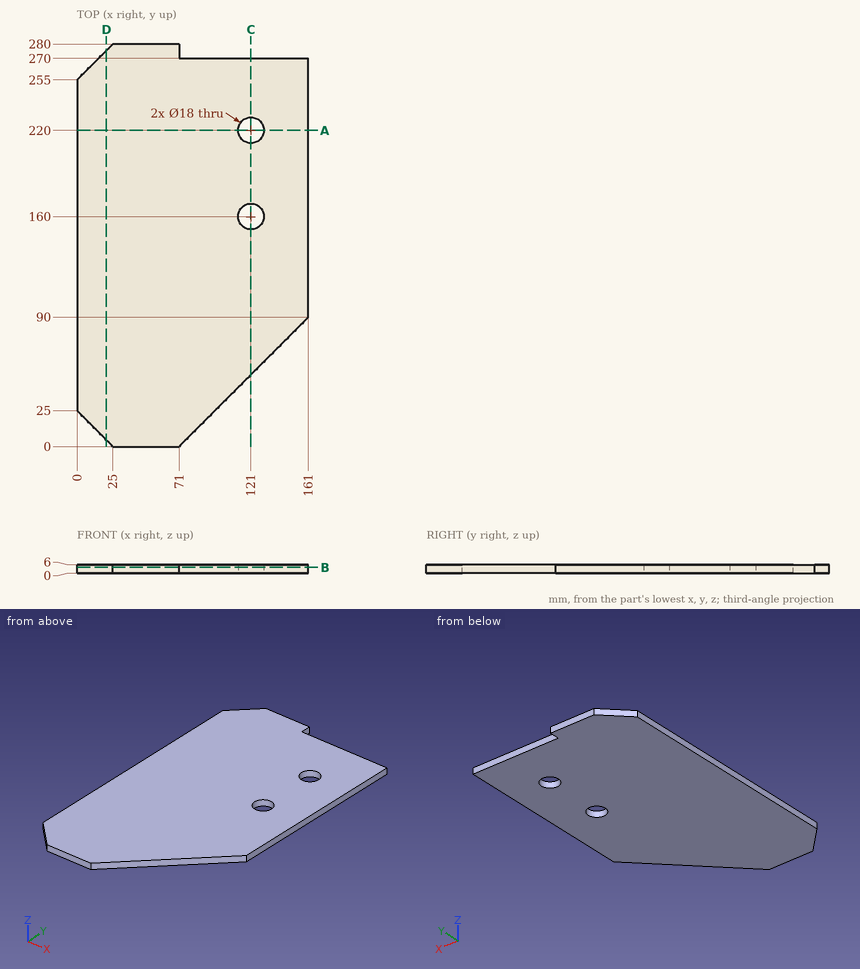
Job drawing, mm, ordinate dimensions from the low corner. One solid piece. Coordinates: 2 decimals unless noted, no trailing zeros. Loops run counter-clockwise (first coordinate to the right, second up) from the corner with the lowest first, then second, coordinate; pieces in that order, holes last. Notation, with made-up numbers: (-2, 56.5) - (31, 56.5) arc R19 ccw to (31, 83.5) - close; hole circle Ø1 at (34.5, -27). An arc over 180 degrees is marked (long way). Write item = value, one per line. Start each with the question number.
Q1. Cut at C-C, the plane x = 121. List the corners of the cut face in (y, z).
Q2. Flat gauge pins, fed straight in: pin 1 Ø10 at (x, y) = (75.5, 71.5) entering from -Z; pin 2 Ø3 at (x, z) = (145, 3) entering from +Y; pin 3 Ø14.5 at (x, y) = (121, 160) entering from +Z. Where does each tip first touch, or does it go through?
Q3. Cut at B-B, the plane z = 3.95. List the corners of the cut face in (x, y), then the cut area to 3 significant figures.
Q4. Cut at D-D, the plane x = 20.5. List the corners of the cut face in (y, z).
Q5. Cut at A-A, the plane y = 220. List the corners of the cut face in (x, z), then the cut area to 3 significant figures.
Q6. Drill centre lines: L1, parallel to X at y = 220, z = 1.9; L2, parallel to Y at x = 119, z = 3.25; L3, parallel to Y at x = 121, z = 2.3. Where is each one in solid material? Low to high.
Computed:
q1.outline = (50, 0) - (151, 0) - (151, 6) - (50, 6) - close; (169, 0) - (211, 0) - (211, 6) - (169, 6) - close; (229, 0) - (270, 0) - (270, 6) - (229, 6) - close
q2.pin_1 = 0
q2.pin_2 = 270
q2.pin_3 = through
q3.outline = (0, 25) - (25, 0) - (71, 0) - (161, 90) - (161, 270) - (71, 270) - (71, 280) - (25, 280) - (0, 255) - close; hole circle Ø18 at (121, 160); hole circle Ø18 at (121, 220)
q3.area = 39,000 mm²
q4.outline = (4.5, 0) - (275.5, 0) - (275.5, 6) - (4.5, 6) - close
q5.outline = (0, 0) - (112, 0) - (112, 6) - (0, 6) - close; (130, 0) - (161, 0) - (161, 6) - (130, 6) - close
q5.area = 858 mm²
q6.L1 = 0 to 112, 130 to 161
q6.L2 = 48 to 151.23, 168.77 to 211.23, 228.77 to 270
q6.L3 = 50 to 151, 169 to 211, 229 to 270
